Input: part model. Units: mm. Frame: model coordinates. A direction names the side the tool comes from. Coordinates: 2 decimals unless noted, no trailing zeros. Order: outer loops, then holes, each group sorted by start corner. A loop starts at its lowest first (then second) coordinate and runs counter-clockwise, first axis right, second up.
from build123d import *

# Parameters (mm, degrees)
F0_R     = 5
F3_DEPTH = 16
F4_R     = 1.99999
F5_R     = 1


# Not quite as in the source:
# - a fillet or chamfer is up to 0.001 mm smaller than in the source, because OpenCascade refuses the exact size


with BuildPart() as f2:
    # F1 (on Right) → F2 (revolve)
    with BuildSketch(Plane.YZ):
        with BuildLine():
            Line((0, 8), (0, 9))
            Line((0, 9), (-18, 9))
            ThreePointArc((-18, 9), (-20.8284271247, 7.8284271247), (-22, 5))
            Line((-22, 5), (0, 5))
            Line((0, 5), (6, 5))
            Line((6, 5), (6, 8))
            Line((6, 8), (0, 8))
        make_face()
    revolve(axis=Axis((0, -24.3240110576, 0), (0, -1, 0)))

    # F0 (on Front) → F3 (join)
    with BuildSketch(Plane.XZ):
        Polygon((6.3508529611, 11), (-6.3508529611, 11), (-12.7017059222, 0), (-6.3508529611, -11), (6.3508529611, -11), (12.7017059222, 0), align=None)
        Circle(F0_R, mode=Mode.SUBTRACT)
    extrude(amount=F3_DEPTH)

    # F4 (radius 2 in the source; OpenCascade refuses exactly that, so slightly less here)
    f4_edges = [f2.edges().sort_by_distance(p)[0] for p in [
        (0, -16, -9),
    ]]
    fillet(f4_edges, radius=F4_R)

    # F5
    f5_edges = [f2.edges().sort_by_distance(p)[0] for p in [
        (-6.350853, -8, 11),
        (-12.701706, -8, 0),
        (-6.350853, -8, -11),
        (6.350853, -8, -11),
        (12.701706, -8, 0),
        (6.350853, -8, 11),
    ]]
    fillet(f5_edges, radius=F5_R)


solid = f2.part
Item 1: Cut plane B-B on y = -5.5. Return loops of the section in (x, z).
Response values:
outline: (-12.41, -0.5) - (-6.64, -10.5) arc R1 ccw to (-5.77, -11) - (5.77, -11) arc R1 ccw to (6.64, -10.5) - (12.41, -0.5) arc R1 ccw to (12.41, 0.5) - (6.64, 10.5) arc R1 ccw to (5.77, 11) - (-5.77, 11) arc R1 ccw to (-6.64, 10.5) - (-12.41, 0.5) arc R1 ccw to start; hole circle Ø10 at (0, 0)
Item 2: Access query for faces 5 (the face through (0, -8, -11)), 6 (the face through (7.81, 2.96, -1.73)), 7 (the face through (-7, -16, 9)). Directions: +Z, -Z, +X, -X, +Y, -Y. A direction counts if a zero-diameter tool reaches every point of the face in a straight line with its end or side. Return the directions, or none.
Response values:
face 5: -Z, +X, -X, +Y, -Y
face 6: +Y
face 7: -Y
Item 3: Draft query along X for faces 1 (the face through (4.88, -7.8, -1.08)), 2 (the face through (0, -8, 11)), 3 (the face through (9.567, -7.888, 5.43)), 4 (the face through (-12.547, -8.112, 0.007)). Return one class per face: pulls with the +X half, pulls with the -X half, needs draft (parallel to the pull), parting line crosses it, or undercut.
Response values:
face 1: undercut
face 2: needs draft
face 3: pulls with the +X half
face 4: pulls with the -X half
Item 4: Ray query, probe 1 along X at (y, z) = (-10, 0); probe 2 along Z at (x, y) = (0, -12); probe 3 along Z at (x, y) = (-3.5, -11.75). Return the intervals inside material, ascending.
Response values:
probe 1: x = -12.55 to -5, 5 to 12.55
probe 2: z = -11 to -5, 5 to 11
probe 3: z = -11 to -3.57, 3.57 to 11
Item 5: Pin query (flat end, axial travel): pin 1 Ø1 at (y, z) = (-5, -3) entering from +X; pin 2 Ø6 at (x, y) = (8, -15.5) entering from -Z; pin 3 Ø1 at (y, z) = (0, -5.5) entering from +X; pin 4 Ø1 at (x, z) = (6.5, 1) entering from -Y. Return the tip coordinate at first contact, or that it passes through.
Response values:
pin 1: stops at x = 11.26
pin 2: stops at z = -11
pin 3: stops at x = 9.81
pin 4: stops at y = -21.85
